Design review of the part shown in the three views and the two pictorial views. Dimensions are in mm from the part's minimum x, y and z. A direction names the side the tool comes from. Round coordinates to 2 decimals unless told otherwise and drop trailing zeros. Loops run counter-clockwise (first coordinate to the right, second up) from the corner with the lowest first, then second, coordinate; pieces in that order, holes last.
1) Insertion check: pin 1 (2 mm diameter, centred on x = 6.5, y = 1.5, fed in from +Z). The pin has a flat end and moves straight along its axis. Give the tip position at first contact, or say it passes through.
2) Wall thickness on L1, parallel to X at y = 3, z = 4.5; L2, parallel to X at y = 1.35, z = 4.5; L3, parallel to Y at x = 6.5, z = 3: over which ranges is each line inside the solid? List them lowest first.
3) Mouldability with a two-part tool opening along Z and no side actions: class the marked faces 1, 2, 3 and 4 as pulls with the +Z half, pulls with the -Z half, needs draft (parallel to the pull), parting line crosses it, or undercut.
4) Take a section at D-D (x = 6.75). State the section outline as (y, z) points, then the cut area to 3 significant figures.
5) Take a section at C-C (y = 0.3). State the section outline as (x, z) points.
6) Take a section at B-B (z = 4.5). State the section outline as (x, y) points, then the cut area to 3 significant figures.
7) Tool access review of the marked faces 5 and 6: name each direction out of +Z, -Z, +X, -X, +Y, -Y from which nothing blocks a thin tool from reaching the whole face with its end or side.
8) Take a section at A-A (x = 4.5). State the section outline as (y, z) points.
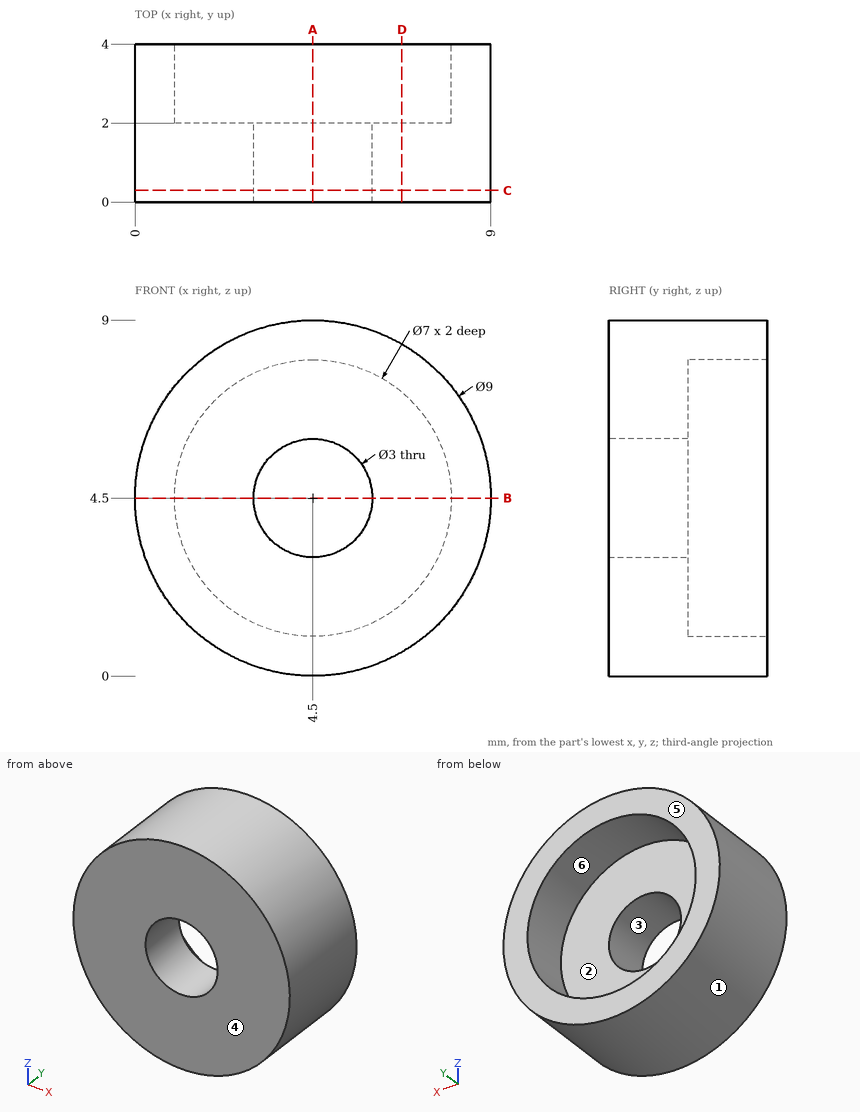
Response:
1. pin 1: stops at z = 8.89
2. L1: x = 0 to 1, 8 to 9
2. L2: x = 0 to 3, 6 to 9
2. L3: y = 0 to 2
3. face 1: parting line crosses it
3. face 2: undercut
3. face 3: undercut
3. face 4: needs draft
4. outline: (0, 0.6) - (4, 0.6) - (4, 1.82) - (2, 1.82) - (2, 7.18) - (4, 7.18) - (4, 8.4) - (0, 8.4) - close
4. area: 20.5 mm2
5. outline: circle Ø9 at (4.5, 4.5); hole circle Ø3 at (4.5, 4.5)
6. outline: (0, 0) - (3, 0) - (3, 2) - (1, 2) - (1, 4) - (0, 4) - close; (6, 0) - (9, 0) - (9, 4) - (8, 4) - (8, 2) - (6, 2) - close
6. area: 16.0 mm2
7. face 5: +Z, -Z, +X, -X, +Y
7. face 6: +Y
8. outline: (0, 0) - (4, 0) - (4, 1) - (2, 1) - (2, 3) - (0, 3) - close; (0, 6) - (2, 6) - (2, 8) - (4, 8) - (4, 9) - (0, 9) - close
